Geometry: final body of the model. Coordinates: model frame, mm. Coordinates: 2 decimals unless noted, no trailing zeros. Write each loop counter-clockwise with the first axis right and the second up, starting at its lowest first coordinate (ties: lowest second). Pieces come first, ordered by that corner, then holes. Notation, with made-up numbers: M 48,83.5 L 104,83.5 A24 cw 104,94.5 Z; hole C -31,5.25 d7. An arc over 180 degrees is marked long. Write item = value, one per line. Start each with the question number.
Item 1: Section C-C on y = 0.75. Output: boundary loops of the cut face in (x, z), plus the area to 3 significant figures.
Item 2: Section A-A on x = 0. Output: boundary loops of the cut face in (y, z).
Item 3: Ray query, L1, parallel to Y at x = 0, z = 13.5; L2, parallel to Z at x = 3.25, y = 3.75; L3, parallel to Y at x = 5.25, z = 15. Return the intervals inside material, ascending. Write a range as [from, to].
Item 4: Section B-B on z = 10. Output: boundary loops of the cut face in (x, y), plus the area to 3 significant figures.
Item 5: Pull-direction query (Y, two-part tool) for faces 1 (the cylindrical face through (-1.56, 7.03, 8.87)), 2 (the flat face through (0.1, 0.1, 0.93)), 3 (the cylindrical face through (-0.54, -2.44, 13.07)), 4 (the flat face through (0, 0, 8)); classes: +Y half, -Y half, draft (parallel to the pull), parting line (faces both ways), or undercut.
Item 6: First-contact query: pin 1 Ø2.5 at (x, y) = (1, 0) entering from +Z; pin 2 Ø5 at (x, y) = (-1, 4.5) entering from -Z; pin 3 Ø6 at (x, y) = (-4, -3.5) entering from -Z. Flat tips, straight axial feed; report the tip coordinate or a pass-through.
Item 7: Section D-D on z = 7.5. Output: boundary loops of the cut face in (x, y), plus the area to 3 significant figures.
Autodesk Inventor part; units mm, degrees
ref_plane "YZ Plane" through (0, 0, 0) normal (1, 0, 0) x (0, 1, 0)
ref_plane "XZ Plane" through (0, 0, 0) normal (0, 1, 0) x (-1, 0, 0)
ref_plane "XY Plane" through (0, 0, 0) normal (0, 0, 1) x (1, 0, 0)
sketch "Sketch1" plane through (0, 0, 0) normal (0, 0, 1) x (1, 0, 0)
  circle A0 centre (0, 0) radius 7.2
  dimension "d0" = 14.4
extrude "Extrusion1" add sketch "Sketch1" along normal blind 18
sketch "Sketch2" plane through (0, 0, 18) normal (0, 0, 1) x (1, 0, 0)
  circle A0 centre (0, 0) radius 2.5
  dimension "d3" = 5
extrude "Extrusion2" cut sketch "Sketch2" against normal blind 10
sketch "Sketch3" plane through (0, 0, 0) normal (0, 0, 1) x (1, 0, 0)
  circle A0 centre (0, 0) radius 7.2
  line L0 (11.2434, 7.2) -> (-13.4853, 7.2) construction
ref_plane "Work Plane1" through (11.2434, 7.2, 0) normal (0, -0.1297, -0.9916) x (-1, 0, 0)
sketch "Sketch4" plane through (11.2434, 7.2, 0) normal (0, -0.1297, -0.9916) x (-1, 0, 0)
  line L0 (30.8181, -24.4459) -> (-8.3313, -24.4459)
  line L1 (-8.3313, -24.4459) -> (-8.3313, 10.1675)
  line L2 (-8.3313, 10.1675) -> (30.8181, 10.1675)
  line L3 (30.8181, 10.1675) -> (30.8181, -24.4459)
  line L4 (30.8181, -24.4459) -> (-8.3313, 10.1675) construction
  line L5 (-8.3313, -24.4459) -> (30.8181, 10.1675) construction
  point P0 (11.2434, -7.1392)
extrude "Extrusion3" cut sketch "Sketch4" along normal blind 10
properties part number "HoleFill3"
Responses:
q1.outline = M -7.16,0.85 L 7.16,0.85 L 7.16,18 L 2.38,18 L 2.38,8 L -2.38,8 L -2.38,18 L -7.16,18 Z
q1.area = 198 mm²
q2.outline = M -7.2,1.89 L 7.2,0 L 7.2,18 L 2.5,18 L 2.5,8 L -2.5,8 L -2.5,18 L -7.2,18 Z
q3.L1 = [-7.2, -2.5], [2.5, 7.2]
q3.L2 = [0.45, 18]
q3.L3 = [-4.93, 4.93]
q4.outline = C 0,0 d14.4; hole C 0,0 d5
q4.area = 143 mm²
q5.face_1 = parting line
q5.face_2 = -Y half
q5.face_3 = undercut
q5.face_4 = undercut
q6.pin_1 = 8
q6.pin_2 = 0.03
q6.pin_3 = 1.01
q7.outline = C 0,0 d14.4
q7.area = 163 mm²
